The model under review builds one solid part; all positions refer to its coordinate system, in mm. A direction names the side the tool comes from. Give positions to 0.01 mm unless a question says otherwise; leave off trailing zeros. Loops run counter-clockwise (first coordinate to the right, second up) from the corner with the lowest first, then second, coordinate; pieces in that order, holes last. Notation, with made-up numbers: M 39,39.25 L 51,39.25 A17 cw 51,71.25 Z; hole C 57,76 d1. An arc over 180 degrees is marked long. Return JSON: item names as keys, results as strings. Group by question number.
```python
from build123d import *

# Parameters (mm, degrees)
SKETCH_1_W          = 15
SKETCH_1_H          = 10
SKETCH_1_W_2        = 12.6
SKETCH_1_H_2        = 7.6
EXTRUDE_1_DEPTH     = 65.5
SKETCH_2_R          = 1.6
CUT_EXTRUDE_1_DEPTH = 65.5


with BuildPart() as part:
    # ｽｹｯﾁ1 → ﾎﾞｽ - 押し出し1 (new, symmetric)
    with BuildSketch(Plane(origin=(0, 0, 0), x_dir=(1, 0, 0), z_dir=(0, 1, 0))):
        Rectangle(SKETCH_1_W, SKETCH_1_H)
        Rectangle(SKETCH_1_W_2, SKETCH_1_H_2, mode=Mode.SUBTRACT)
    extrude(amount=EXTRUDE_1_DEPTH, both=True)

    # ｽｹｯﾁ2 → ｶｯﾄ - 押し出し1 (cut, symmetric)
    with BuildSketch(Plane.ZY.offset(7.5)):
        with Locations((0, 32.5)):
            Circle(SKETCH_2_R)
    cut_extrude_1 = extrude(amount=CUT_EXTRUDE_1_DEPTH, both=True, mode=Mode.SUBTRACT)

    # ﾐﾗｰ1: ｶｯﾄ - 押し出し1 across plane
    add(cut_extrude_1.mirror(Plane.ZX), mode=Mode.SUBTRACT)


solid = part.part
```
(1) Add section A-A (z = 0). Write out the cut boundary in (x, y), and give its area (3 significant figures).
(2) Add section B-B (y = -24). Write out the cut boundary in (x, z), and give its area (3 significant figures).
(3) Add section C-C (x = 0). Write out the cut boundary in (y, z), and give its area (3 significant figures).
(4) For pin 1 (1.9 mm diameter, centred on y = 32.5, z = 0, fed in from +X), flat-tipped, find the tip position at first contact; note if it passes through.
(5) For probe 1 along Y at (x, z) = (6.7, 0); probe 2 along X at (y, z) = (57, 0.5); probe 3 along Z at (x, y) = (-1, -12), list the stretches that pass through material, from the lowest coordinate up.
(6) For faces 4 (the cylindrical face through (6.89, -30.94, -0.35)), 5 (the flat face through (-6.3, 1, 0)), list the 3-axis set-ups (+Z, -Z, +X, -X, +Y, -Y) from which the entire face can be reached by the end or side of a thin tool; tool diameter is ignored.
(7) Mouldability with a two-part tool opening along Y and no side actions: class faces 1 (the cylindrical face through (6.89, 30.94, -0.35)), 2 (the flat face through (0, 1, -3.8)), 3 (the flat face through (0, 65.5, 4)) as released by +Y, released by -Y, zero draft, split by the parting line, or undercut.
Verdict:
{
 "1": {"outline": "M -7.5,-65.5 L -6.3,-65.5 L -6.3,-34.1 L -7.5,-34.1 Z; M -7.5,-30.9 L -6.3,-30.9 L -6.3,30.9 L -7.5,30.9 Z; M -7.5,34.1 L -6.3,34.1 L -6.3,65.5 L -7.5,65.5 Z; M 6.3,-65.5 L 7.5,-65.5 L 7.5,-34.1 L 6.3,-34.1 Z; M 6.3,-30.9 L 7.5,-30.9 L 7.5,30.9 L 6.3,30.9 Z; M 6.3,34.1 L 7.5,34.1 L 7.5,65.5 L 6.3,65.5 Z", "area": "299 mm²"},
 "2": {"outline": "M -7.5,-5 L 7.5,-5 L 7.5,5 L -7.5,5 Z; hole M -6.3,-3.8 L 6.3,-3.8 L 6.3,3.8 L -6.3,3.8 Z", "area": "54.2 mm²"},
 "3": {"outline": "M -65.5,-5 L 65.5,-5 L 65.5,-3.8 L -65.5,-3.8 Z; M -65.5,3.8 L 65.5,3.8 L 65.5,5 L -65.5,5 Z", "area": "314 mm²"},
 "4": {"pin 1": "passes through"},
 "5": {"probe 1": "y = -65.5 to -34.1, -30.9 to 30.9, 34.1 to 65.5", "probe 2": "x = -7.5 to -6.3, 6.3 to 7.5", "probe 3": "z = -5 to -3.8, 3.8 to 5"},
 "6": {"face 4": "+X, -X", "face 5": "+Y, -Y"},
 "7": {"face 1": "undercut", "face 2": "zero draft", "face 3": "released by +Y"}
}
